Build history of the part. All positions in model axes, mm. A direction names the side the tool comes from. Give positions to 0.01 mm unless a question says otherwise; leave off trailing zeros. Loops run counter-clockwise (first coordinate to the right, second up) from the corner with the lowest first, then second, coordinate; pieces in that order, holes last. Notation, with made-up numbers: (86, 50) - (108, 50) arc R16 cw to (108, 69) - close; hole circle Ø3 at (82, 81.5). An arc over 180 degrees is marked (long way). Return JSON: item names as keys, results as strings. Group by question number.
1) Slice it at A-A (x = 0). List the corners of the cut face in (y, z), and give its area (3 significant figures).
2) Drill centre lines: probe 1 along Z at (x, y) = (0, -1.75); probe 2 along X at (y, z) = (0.5, 10); probe 3 along Z at (x, y) = (0, 0). Where is each one in solid material? Low to high. Write a range as from..to.
3) Slice it at B-B (z = 12.5). List the corners of the cut face in (x, y), and give its area (3 significant figures).
4) Slice it at C-C (z = 10). List the corners of the cut face in (x, y), and give its area (3 significant figures).
5) Mould opens along Y. For faces 1 (the face through (0, 0, 14.5)), 2 (the face through (0, 0, 3)) say: released by +Y, released by -Y, zero draft, split by the parting line, or undercut.
6) 3-axis set-ups, long thin cutter, end or side, ignore diameter. For faces 3 (the face through (0, -1, 0)), 4 (the face through (0, -0.5, 1)): which of +Z, -Z, +X, -X, +Y, -Y reach the whole face in a straight line?
7) Drop flat-ended pins along their axis: pin 1 (5 mm diameter, centred on x = 2.5, z = 12.5, fed in from +Y); pin 2 (0.9 mm diameter, centred on x = 0.5, z = 2, fed in from +Y); pin 3 (0.8 mm diameter, centred on x = 1, y = 0, fed in from -Z). Give the stop position or say it passes through.
```python
from build123d import *

# Parameters (mm, degrees)
F1_DEPTH = 14.5
F2_DEPTH = 4
F3_DEPTH = 3
F5_R     = 3.1
F6_DEPTH = 10.751
F7_R     = 3
F9_R     = 1.3


# Not quite as in the source:
# - a fillet or chamfer that OpenCascade refuses, or shapes differently, is made with other operations: its cross-section is extruded or revolved along the edge and cut away or added


with BuildPart() as f1:
    # F0 (on Top) → F1 (new body)
    with BuildSketch(Plane.XY):
        with BuildLine():
            Line((-4.3714985989, 0.5), (4.3714985989, 0.5))
            ThreePointArc((4.3714985989, 0.5), (0, 4.4), (-4.3714985989, 0.5))
        make_face()
        with BuildLine():
            ThreePointArc((4.3714985989, -0.5), (4.392868871, -0.2504058355), (4.4, 0))
            ThreePointArc((4.4, 0), (4.392868871, 0.2504058355), (4.3714985989, 0.5))
            Line((4.3714985989, 0.5), (-4.3714985989, 0.5))
            ThreePointArc((-4.3714985989, 0.5), (-4.4, 0), (-4.3714985989, -0.5))
            Line((-4.3714985989, -0.5), (4.3714985989, -0.5))
        make_face()
        with BuildLine():
            ThreePointArc((-4.3714985989, -0.5), (0, -4.4), (4.3714985989, -0.5))
            Line((4.3714985989, -0.5), (-4.3714985989, -0.5))
        make_face()
    extrude(amount=F1_DEPTH)

    # F0 (on Top) → F2 (join)
    with BuildSketch(Plane.XY):
        with BuildLine():
            ThreePointArc((-4.3714985989, -0.5), (-4.4, 0), (-4.3714985989, 0.5))
            Line((-4.3714985989, 0.5), (-5.9791303716, 0.5))
            ThreePointArc((-5.9791303716, 0.5), (-6, 0), (-5.9791303716, -0.5))
            Line((-5.9791303716, -0.5), (-4.3714985989, -0.5))
        make_face()
        with BuildLine():
            Line((5.9791303716, -0.5), (4.3714985989, -0.5))
            ThreePointArc((4.3714985989, -0.5), (0, -4.4), (-4.3714985989, -0.5))
            Line((-4.3714985989, -0.5), (-5.9791303716, -0.5))
            ThreePointArc((-5.9791303716, -0.5), (0, -6), (5.9791303716, -0.5))
        make_face()
        with BuildLine():
            ThreePointArc((4.3714985989, 0.5), (4.392868871, 0.2504058355), (4.4, 0))
            ThreePointArc((4.4, 0), (4.392868871, -0.2504058355), (4.3714985989, -0.5))
            Line((4.3714985989, -0.5), (5.9791303716, -0.5))
            ThreePointArc((5.9791303716, -0.5), (5.9947803225, -0.2502176759), (6, 0))
            ThreePointArc((6, 0), (5.9947803225, 0.2502176759), (5.9791303716, 0.5))
            Line((5.9791303716, 0.5), (4.3714985989, 0.5))
        make_face()
        with BuildLine():
            ThreePointArc((-4.3714985989, 0.5), (0, 4.4), (4.3714985989, 0.5))
            Line((4.3714985989, 0.5), (5.9791303716, 0.5))
            ThreePointArc((5.9791303716, 0.5), (0, 6), (-5.9791303716, 0.5))
            Line((-5.9791303716, 0.5), (-4.3714985989, 0.5))
        make_face()
    extrude(amount=F2_DEPTH)

    # F0 (on Top) → F3 (cut)
    with BuildSketch(Plane.XY):
        with BuildLine():
            ThreePointArc((-4.3714985989, -0.5), (-4.4, 0), (-4.3714985989, 0.5))
            Line((-4.3714985989, 0.5), (-5.9791303716, 0.5))
            ThreePointArc((-5.9791303716, 0.5), (-6, 0), (-5.9791303716, -0.5))
            Line((-5.9791303716, -0.5), (-4.3714985989, -0.5))
        make_face()
        with BuildLine():
            ThreePointArc((4.3714985989, -0.5), (4.392868871, -0.2504058355), (4.4, 0))
            ThreePointArc((4.4, 0), (4.392868871, 0.2504058355), (4.3714985989, 0.5))
            Line((4.3714985989, 0.5), (-4.3714985989, 0.5))
            ThreePointArc((-4.3714985989, 0.5), (-4.4, 0), (-4.3714985989, -0.5))
            Line((-4.3714985989, -0.5), (4.3714985989, -0.5))
        make_face()
        with BuildLine():
            ThreePointArc((4.3714985989, 0.5), (4.392868871, 0.2504058355), (4.4, 0))
            ThreePointArc((4.4, 0), (4.392868871, -0.2504058355), (4.3714985989, -0.5))
            Line((4.3714985989, -0.5), (5.9791303716, -0.5))
            ThreePointArc((5.9791303716, -0.5), (5.9947803225, -0.2502176759), (6, 0))
            ThreePointArc((6, 0), (5.9947803225, 0.2502176759), (5.9791303716, 0.5))
            Line((5.9791303716, 0.5), (4.3714985989, 0.5))
        make_face()
    extrude(amount=F3_DEPTH, mode=Mode.SUBTRACT)

    # F5 (on offset) → F6 (cut, through all)
    with BuildSketch(Plane.XZ.offset(4.75)):
        with Locations((0, 10)):
            Circle(F5_R)
    extrude(amount=-F6_DEPTH, mode=Mode.SUBTRACT)

    # F7
    f7_edges = [f1.edges().sort_by_distance(p)[0] for p in [
        (0, 6, 0),
        (0, -6, 0),
    ]]
    fillet(f7_edges, radius=F7_R)

    # F8: fillet of radius 1.7 on 1 edges, made by hand

    # F8_s1 → F8_t2 (revolve, cut)
    with BuildSketch(Plane(origin=(0, 0, 0), x_dir=(0, 0, 1), z_dir=(0.0833333333, -0.9965217286, 0))):
        with BuildLine():
            ThreePointArc((3, -6), (3.7282856857, -5.3727611072), (4, -4.4508066615))
            Line((4, -4.4508066615), (4.034, -4.4508066615))
            Line((4.034, -4.4508066615), (4.034, -6))
            Line((4.034, -6), (4, -6.034))
            ThreePointArc((4, -6.034), (3.5, -6.034), (3.014, -6.0309838668))
            Line((3.014, -6.0309838668), (3, -6))
        make_face()
    revolve(axis=Axis((0, 0, 4), (0, 0, 1)), mode=Mode.SUBTRACT)

    # F9
    f9_edges = [f1.edges().sort_by_distance(p)[0] for p in [
        (4.371499, 0.5, 14.5),
    ]]
    fillet(f9_edges, radius=F9_R)


solid = f1.part
```
Results:
{
 "1": {"outline": "(-6, 3) arc R3 ccw to (-3, 0) - (-0.5, 0) - (-0.5, 3) - (0.5, 3) - (0.5, 0) - (3, 0) arc R3 ccw to (6, 3) arc R1.7 ccw to (4.45, 4) - (4.4, 4) - (4.4, 6.9) - (-4.4, 6.9) - (-4.4, 4) - (-4.45, 4) arc R1.7 ccw to start; (-4.4, 13.1) - (4.4, 13.1) - (4.4, 13.2) arc R1.3 ccw to (3.1, 14.5) - (-3.1, 14.5) arc R1.3 ccw to (-4.4, 13.2) - close", "area": "77.4 mm2"},
 "2": {"probe 1": "0..6.9, 13.1..14.5", "probe 2": "-4.37..-3.1, 3.1..4.37", "probe 3": "3..6.9, 13.1..14.5"},
 "3": {"outline": "(-1.83, -4) - (-1.83, 4) arc R4.4 ccw to start; (1.83, -4) arc R4.4 ccw to (1.83, 4) - close", "area": "29.5 mm2"},
 "4": {"outline": "(-3.1, -3.12) - (-3.1, 3.12) arc R4.4 ccw to start; (3.1, -3.12) arc R4.4 ccw to (3.1, 3.12) - close", "area": "11.2 mm2"},
 "5": {"face 1": "zero draft", "face 2": "undercut"},
 "6": {"face 3": "-Z, +X, -X, +Y, -Y", "face 4": "-Z, +X, -X"},
 "7": {"pin 1": "y = 4.4", "pin 2": "y = 5.93", "pin 3": "z = 3"}
}
